```python
from build123d import *

# Parameters (mm, degrees)
F0_R     = 27.5
F1_DEPTH = 45
F2_R     = 41.570783
F2_R_2   = 26.5
F3_DEPTH = 43
F4_R     = 10.25
F5_DEPTH = 45.001
F7_DEPTH = 45.001


with BuildPart() as f1:
    # F0 (on Top) → F1 (new body)
    with BuildSketch(Plane.XY):
        Circle(F0_R)
    extrude(amount=F1_DEPTH)

    # F2 (on face) → F3 (cut)
    with BuildSketch(Plane.XY.offset(45)):
        Circle(F2_R)
        Circle(F2_R_2, mode=Mode.SUBTRACT)
    extrude(amount=-F3_DEPTH, mode=Mode.SUBTRACT)

    # F4 (on face) → F5 (cut, through all)
    with BuildSketch(Plane.XY.offset(45)):
        Circle(F4_R)
    extrude(amount=-F5_DEPTH, mode=Mode.SUBTRACT)

    # F6 (on face) → F7 (cut, through all)
    with BuildSketch(Plane.XY.offset(45)):
        with BuildLine():
            ThreePointArc((-5.25, 10.231691), (0, 11.5), (5.25, 10.231691))
            Line((5.25, 10.231691), (11.822918, 22.593552))
            ThreePointArc((11.822918, 22.593552), (0, 25.5), (-11.822918, 22.593552))
            Line((-11.822918, 22.593552), (-5.25, 10.231691))
        make_face()
        with BuildLine():
            ThreePointArc((-11.485904, 0.569212), (-9.959292, 5.75), (-6.235904, 9.662479))
            Line((-6.235904, 9.662479), (-13.655131, 21.535724))
            ThreePointArc((-13.655131, 21.535724), (-22.083648, 12.75), (-25.478049, 1.057829))
            Line((-25.478049, 1.057829), (-11.485904, 0.569212))
        make_face()
        with BuildLine():
            ThreePointArc((-6.235904, -9.662479), (-9.959292, -5.75), (-11.485904, -0.569212))
            Line((-11.485904, -0.569212), (-25.478049, -1.057829))
            ThreePointArc((-25.478049, -1.057829), (-22.083648, -12.75), (-13.655131, -21.535724))
            Line((-13.655131, -21.535724), (-6.235904, -9.662479))
        make_face()
        with BuildLine():
            ThreePointArc((5.25, -10.231691), (0, -11.5), (-5.25, -10.231691))
            Line((-5.25, -10.231691), (-11.822918, -22.593552))
            ThreePointArc((-11.822918, -22.593552), (0, -25.5), (11.822918, -22.593552))
            Line((11.822918, -22.593552), (5.25, -10.231691))
        make_face()
        with BuildLine():
            ThreePointArc((11.485904, -0.569212), (9.959292, -5.75), (6.235904, -9.662479))
            Line((6.235904, -9.662479), (13.655131, -21.535724))
            ThreePointArc((13.655131, -21.535724), (22.083648, -12.75), (25.478049, -1.057829))
            Line((25.478049, -1.057829), (11.485904, -0.569212))
        make_face()
        with BuildLine():
            ThreePointArc((6.235904, 9.662479), (9.959292, 5.75), (11.485904, 0.569212))
            Line((11.485904, 0.569212), (25.478049, 1.057829))
            ThreePointArc((25.478049, 1.057829), (22.083648, 12.75), (13.655131, 21.535724))
            Line((13.655131, 21.535724), (6.235904, 9.662479))
        make_face()
    extrude(amount=-F7_DEPTH, mode=Mode.SUBTRACT)


solid = f1.part
```
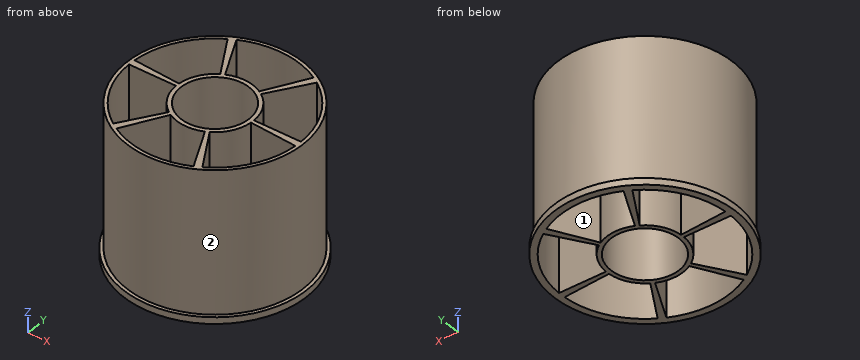
Input: part model. Units: mm. Frame: model coordinates. Face numbers are marked on the shaded views. Round coordinates to 2 decimals unless told otherwise and drop trailing zeros. Loops run counter-clockwise (first coordinate to the right, second up) from the corner with the lowest first, then second, coordinate; pieces in that order, holes last.
1) Section query B-B on z = 8. Return the cut outline in (x, y).
Ans:
outline: circle Ø53 at (0, 0); hole (-25.48, -1.06) arc R25.5 ccw to (-13.66, -21.54) - (-6.24, -9.66) arc R11.5 cw to (-11.49, -0.57) - close; hole (-25.48, 1.06) - (-11.49, 0.57) arc R11.5 cw to (-6.24, 9.66) - (-13.66, 21.54) arc R25.5 ccw to start; hole (-11.82, -22.59) arc R25.5 ccw to (11.82, -22.59) - (5.25, -10.23) arc R11.5 cw to (-5.25, -10.23) - close; hole (-11.82, 22.59) - (-5.25, 10.23) arc R11.5 cw to (5.25, 10.23) - (11.82, 22.59) arc R25.5 ccw to start; hole circle Ø20.5 at (0, 0); hole (6.24, -9.66) - (13.66, -21.54) arc R25.5 ccw to (25.48, -1.06) - (11.49, -0.57) arc R11.5 cw to start; hole (6.24, 9.66) arc R11.5 cw to (11.49, 0.57) - (25.48, 1.06) arc R25.5 ccw to (13.66, 21.54) - close
2) Section query C-C on y = 5. Return the cut outline in (x, z) (3 decimals).
Ans:
outline: (-27.042, 0) - (-25.005, 0) - (-25.005, 45) - (-26.024, 45) - (-26.024, 2) - (-27.042, 2) - close; (-10.356, 0) - (-8.948, 0) - (-8.948, 45) - (-10.356, 45) - close; (8.948, 0) - (10.356, 0) - (10.356, 45) - (8.948, 45) - close; (25.005, 0) - (27.042, 0) - (27.042, 2) - (26.024, 2) - (26.024, 45) - (25.005, 45) - close
3) Section query A-A on x = 0. Return the cut outline in (y, z), plus the area to 4 significant figures.
Ans:
outline: (-27.5, 0) - (-25.5, 0) - (-25.5, 45) - (-26.5, 45) - (-26.5, 2) - (-27.5, 2) - close; (-11.5, 0) - (-10.25, 0) - (-10.25, 45) - (-11.5, 45) - close; (10.25, 0) - (11.5, 0) - (11.5, 45) - (10.25, 45) - close; (25.5, 0) - (27.5, 0) - (27.5, 2) - (26.5, 2) - (26.5, 45) - (25.5, 45) - close
area: 206.5 mm2
4) Section query D-D on x = -9.5. Return the cut outline in (y, z).
Ans:
outline: (-25.81, 0) - (-23.66, 0) - (-23.66, 45) - (-24.74, 45) - (-24.74, 2) - (-25.81, 2) - close; (-18.22, 0) - (-14.89, 0) - (-14.89, 45) - (-18.22, 45) - close; (-6.48, 0) - (-3.85, 0) - (-3.85, 45) - (-6.48, 45) - close; (3.85, 0) - (6.48, 0) - (6.48, 45) - (3.85, 45) - close; (14.89, 0) - (18.22, 0) - (18.22, 45) - (14.89, 45) - close; (23.66, 0) - (25.81, 0) - (25.81, 2) - (24.74, 2) - (24.74, 45) - (23.66, 45) - close
5) Pin query (flat end, axial travel): pin 1 (10 mm diameter, centred on y = 0.5, z = 7.5, fed in from -X); pin 2 (2 mm diameter, centred on x = -13, z = 40.5, fed in from +Y); pin 3 (10 mm diameter, centred on x = -9.5, z = 16, fed in from +Y); pin 4 (16.5 mm diameter, centred on x = 0, y = 0, fed in from -Z). Return the tip coordinate at first contact, or that it passes through.
Ans:
pin 1: stops at x = -26.5
pin 2: stops at y = 23.63
pin 3: stops at y = 26.12
pin 4: passes through
6) Material intervals for line 1 (X direction, y = -17.5, z = 42.5); line 2 (Y direction, x = 16.5, z = 16); line 3 (X direction, y = -20, z = 13.5), sorted ascending.
Ans:
line 1: x = -19.9 to -18.55, -11.13 to -9.11, 9.11 to 11.13, 18.55 to 19.9
line 2: y = -20.74 to -19.44, -0.74 to 0.74, 19.44 to 20.74
line 3: x = -17.39 to -15.82, -12.7 to -10.44, 10.44 to 12.7, 15.82 to 17.39
7) Pull-direction query (X, two-part tool) for the marked faces 1 and 2; classes: released by +X, released by -X, zero draft, split by the parting line, or undercut.
Ans:
face 1: undercut
face 2: split by the parting line
